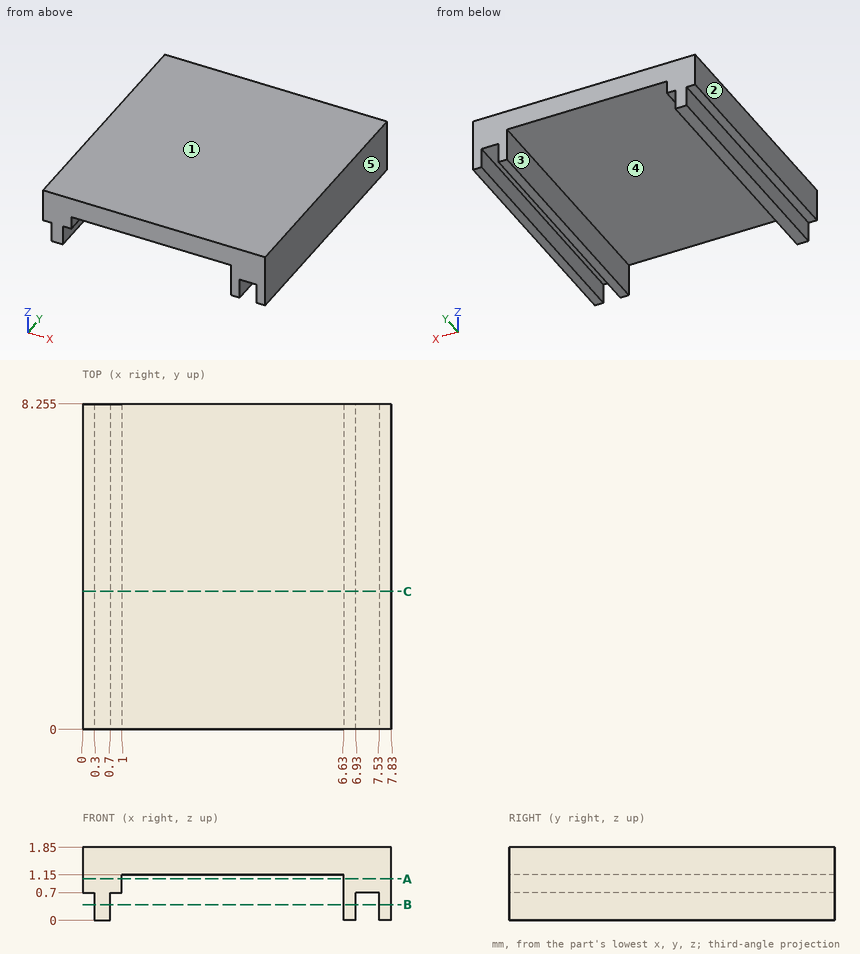
Can you work these out from the drawing? Everything is in mm from the part's minimum corner. A direction names the side the tool comes from. Coordinates: 2 decimals unless noted, no trailing zeros. Order: outer loops, then holes, each group sorted by start corner. A loop starts at its lowest first (then second) coordinate and runs counter-clockwise, first axis right, second up. Notation, with made-up numbers: (-16.5, 11) -> (-6.5, 11) arc R14 ccw to (-6.5, 32) -> close; hole circle Ø9 at (-0.75, 81.25). An arc over 180 degrees is marked (long way). Return JSON: item names as keys, results as strings.
1) If we section it at A-A on z = 1.05: List the corners of the cut face in (x, y) for me (1 decimal).
Conclusion:
{"outline": "(0, 0) -> (1, 0) -> (1, 8.3) -> (0, 8.3) -> close; (6.6, 0) -> (7.8, 0) -> (7.8, 8.3) -> (6.6, 8.3) -> close"}
2) If I drill on probe 1 along X at (y, z) = (1.25, 0.5); probe 2 along X at (y, z) = (4.5, 0.8); probe 3 along Z at (x, y) = (2.25, 7), over which ranges is the centre line in solid material (lowest first)?
Conclusion:
{"probe 1": "x = 0.3 to 0.7, 6.63 to 6.93, 7.53 to 7.83", "probe 2": "x = 0 to 1, 6.63 to 7.83", "probe 3": "z = 1.15 to 1.85"}
3) I'm going to push flat-ended pins straight in: P1, Ø1, axis at x = 3.5, z = 1, coming from the +Y side (3 decimals); P2, Ø3, axis at x = 3.5, y = 5, coming from the -Z side. Where does each tip first touch, or does it pass through?
Conclusion:
{"P1": "stops at y = 8.255", "P2": "stops at z = 1.15"}
4) On a 3-axis mill with a long thin cutter (end or side, diameter ignored), from which of +Z, -Z, +X, -X, +Y, -Y can I reach the whole of each face in a straight line? I mean the marked faces 4 and 5. Say none if no direction works.
Conclusion:
{"face 4": "-Z, +Y, -Y", "face 5": "+Z, -Z, +X, +Y, -Y"}
5) If we section it at B-B on z = 0.4: State how many separate pieces and enclosed holes the cut face has.
Conclusion:
{"separate pieces": "3", "enclosed holes": "0"}
6) If we section it at C-C on y = 3.5: List the corners of the cut face in (x, z) for me.
Conclusion:
{"outline": "(0, 0.7) -> (0.3, 0.7) -> (0.3, 0) -> (0.7, 0) -> (0.7, 0.7) -> (1, 0.7) -> (1, 1.15) -> (6.63, 1.15) -> (6.63, 0) -> (6.93, 0) -> (6.93, 0.7) -> (7.53, 0.7) -> (7.53, 0) -> (7.83, 0) -> (7.83, 1.85) -> (0, 1.85) -> close"}
7) Thinking about a two-plate mould opening in X: for the marked faces 1, 2 and 3, which applies, +X half, -X half, draft (parallel to the pull), parting line (faces both ways), or undercut?
Conclusion:
{"face 1": "draft", "face 2": "-X half", "face 3": "undercut"}
